from build123d import *

# Parameters (mm, degrees)
FILLET085_R          = 6
POCKET030_DEPTH      = 135.001
POCKET030_DEPTH_BACK = 135.001
POCKET031_DEPTH      = 135.001
POCKET031_DEPTH_BACK = 135.001


with BuildPart() as part:
    # Sketch170 → Revolution088 (revolve)
    with BuildSketch(Plane.XY):
        with BuildLine():
            Line((0, -29.430492), (0, -256.067871))
            add(Edge.make_bspline(
                [(118.087006, -247.149109), (78.943573, -254.209778), (41.881203, -256.067871), (0, -256.067871)],
                knots=[0, 0, 0, 0, 1, 1, 1, 1], degree=3))
            add(Edge.make_bspline(
                [(0, -29.430492), (51.371703, -29.430492), (85.484656, -26.492154), (104.24503, -87.257226), (119.255189, -159.347806), (118.910339, -227.073486), (118.087006, -247.149109)],
                knots=[0, 0, 0, 0, 0.25, 0.5, 0.75, 1, 1, 1, 1], degree=3))
        make_face()
    revolve(axis=Axis((0, 0, 0), (0, 1, 0)))

    # Sketch171 → Groove082 (revolve, cut)
    with BuildSketch(Plane.XY):
        with BuildLine():
            Line((0, 75), (0, -75))
            ThreePointArc((0, -75), (75, 0), (0, 75))
        make_face()
    revolve(axis=Axis((0, 0, 0), (0, 1, 0)), mode=Mode.SUBTRACT)

    # Fillet085
    fillet085_edges = [part.edges().sort_by_distance(p)[0] for p in [
        (-67.994287, -31.650859, 0),
    ]]
    fillet(fillet085_edges, radius=FILLET085_R)

    # Sketch172 → Groove083 (revolve, cut)
    with BuildSketch(Plane.XY):
        with BuildLine():
            Line((15, -298), (135, -298))
            ThreePointArc((135, -298), (75, -238), (15, -298))
        make_face()
        with BuildLine():
            Line((-135, -298), (-15, -298))
            ThreePointArc((-15, -298), (-75, -238), (-135, -298))
        make_face()
    revolve(axis=Axis((15, -298, 0), (1, 0, 0)), mode=Mode.SUBTRACT)

    # Sketch172 → Revolution089 (revolve)
    with BuildSketch(Plane.XY):
        with BuildLine():
            Line((15, -298), (135, -298))
            ThreePointArc((135, -298), (75, -238), (15, -298))
        make_face()
        with BuildLine():
            Line((-135, -298), (-15, -298))
            ThreePointArc((-15, -298), (-75, -238), (-135, -298))
        make_face()
    revolve(axis=Axis((15, -298, 0), (1, 0, 0)))

    # Sketch173 → Pocket030 (cut, two sides)
    with BuildSketch(Plane.YZ) as pocket030_sk:
        Polygon((-309.733459, 84.757393), (-36.255981, 111.745285), (-36.255981, 192.709015), (-309.733459, 192.709015), align=None)
    extrude(amount=-POCKET030_DEPTH, mode=Mode.SUBTRACT)
    extrude(pocket030_sk.sketch, amount=POCKET030_DEPTH_BACK, mode=Mode.SUBTRACT)

    # Sketch174 → Pocket031 (cut, two sides)
    with BuildSketch(Plane.YZ) as pocket031_sk:
        Polygon((-276.336304, -71.472351), (-109.323242, -126.410881), (-109.323242, -220.905121), (-276.336304, -220.905121), align=None)
    extrude(amount=-POCKET031_DEPTH, mode=Mode.SUBTRACT)
    extrude(pocket031_sk.sketch, amount=POCKET031_DEPTH_BACK, mode=Mode.SUBTRACT)


with BuildPart() as part_1:
    # Body051 placement: moved
    add(part.part.moved(Location((0, 1197.018312, 0.388141))))


solid = part_1.part
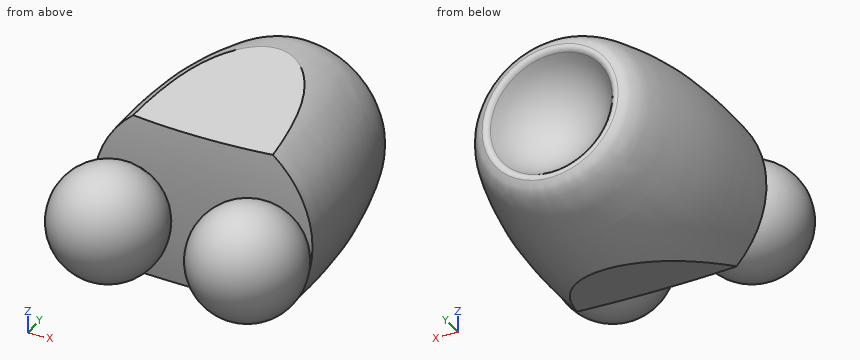
For this review, take the finished solid that the model builds, in its own axes (mm). Give positions to 0.01 mm unless a question says otherwise; leave off trailing zeros. Order: outer loops, then holes, each group sorted by start corner. A loop starts at its lowest first (then second) coordinate and runs counter-clockwise, first axis right, second up. Notation, with made-up numbers: M 14.25,21 L 25.25,21 A22 ccw 25.25,35 Z; hole C -38,81.25 d11. An arc over 180 degrees is marked long. Answer in a Markdown table with one row per item. Add a question column.
(1) Consider section B-B on y = 864. State the section outline as (x, z) points, and give its area (3 significant figures).
(2) Wall thickness on probe 1 along Y at (x, z) = (-41, -45); probe 2 along X at (y, z) = (855.5, -32.5); probe 3 along X at (y, z) = (893, -13): over which ranges is each line inside the solid? List them lowest first. Write a range as [from, to].
(3) Consider section A-A on z = 46.5. Give the number of separate pieces and of enclosed holes in the cut face, and give its area (3 significant figures).
(4) For pin 1 (3 mm diameter, centred on x = -74, y = 1078.5, fed in from -Z); pin 2 (6 mm diameter, centred on x = -71.5, z = -12.5, fed in from -Y); pin 3 (1.5 mm diameter, centred on x = -30.5, z = -43.5, fed in from -Y), all flat-tipped, find the tip position at first contact; note any pin that passes through.
Evaluation:
| question | item | result |
|---|---|---|
| 1 | outline | C -75,0.39 d97.44; C 75,0.39 d97.44 |
| 1 | area | 14,900 mm^2 |
| 2 | probe 1 | y = [879.42, 918.61], [942.84, 1153.61] |
| 2 | probe 2 | x = [-99.99, -50.01], [50.01, 99.99] |
| 2 | probe 3 | x = [-133.18, -16.82], [16.82, 133.18] |
| 3 | separate pieces | 3 |
| 3 | enclosed holes | 0 |
| 3 | area | 51,000 mm^2 |
| 4 | pin 1 | stops at z = -82.77 |
| 4 | pin 2 | stops at y = 839.92 |
| 4 | pin 3 | stops at y = 942.29 |
